Input: dimensioned drawing with shaded views. Units: mm. Origin: part minimum x, y, z. Round coordinates to 2 decimals unless told otherwise and drop trailing zeros. Order: outer loops, then holes, each group sorted by start corner. A loop starts at its lowest first (then second) coordinate and runs counter-clockwise, first axis right, second up. Notation, with made-up numbers: M 10.25,53.5 L 58.25,53.5 A22 ccw 58.25,85.5 Z; hole C -26,-8.5 d10. An arc over 180 degrees is marked long. Put each result on its own line as item: value. Start each with the question number.
1) Section B-B, the plane x = 107. Return loops of the section in (y, z), then the cut area to 3 significant figures.
2) Material intervals for probe 1 along Y at (x, z) = (8, 1.3); probe 2 along X at (y, z) = (162, 0.7); probe 3 along X at (y, z) = (34, 2.5), sorted ascending. Write a range as [from, to].
3) Section A-A, the plane z = 2.45. Return loops of the section in (x, y).
4) First-contact query: P1, Ø3, axis at x = 152, y = 162, coming from the +Z side. Flat tip, straight axial feed; report the tip coordinate or a pass-through.
5) Section C-C, the plane y = 135. Return loops of the section in (x, z).
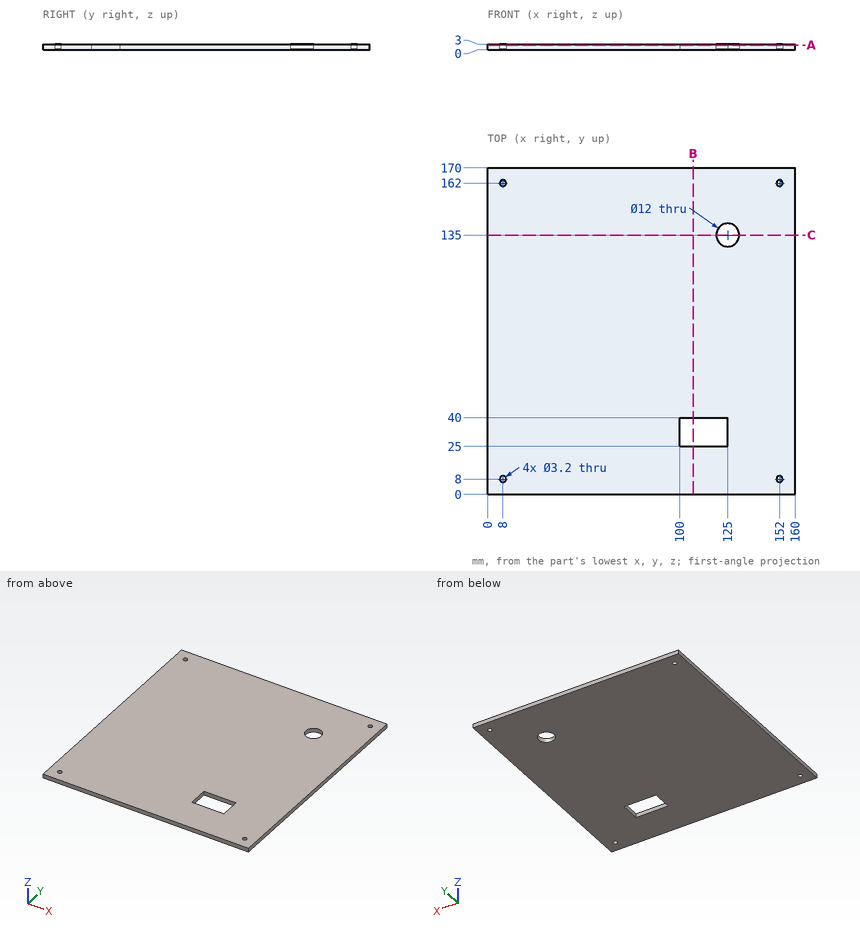
Result sheet:
1. outline: M 0,0 L 25,0 L 25,3 L 0,3 Z; M 40,0 L 170,0 L 170,3 L 40,3 Z
1. area: 465 mm2
2. probe 1: y = [0, 6.4], [9.6, 160.4], [163.6, 170]
2. probe 2: x = [0, 6.4], [9.6, 150.4], [153.6, 160]
2. probe 3: x = [0, 100], [125, 160]
3. outline: M 0,0 L 160,0 L 160,170 L 0,170 Z; hole C 8,8 d3.2; hole C 8,162 d3.2; hole M 100,25 L 125,25 L 125,40 L 100,40 Z; hole C 125,135 d12; hole C 152,8 d3.2; hole C 152,162 d3.2
4. P1: passes through
5. outline: M 0,0 L 119,0 L 119,3 L 0,3 Z; M 131,0 L 160,0 L 160,3 L 131,3 Z
